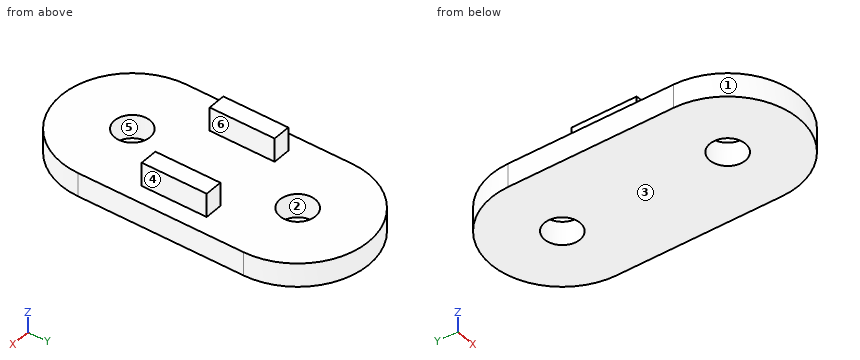
```python
from build123d import *

# Parameters (mm, degrees)
SKETCH_R     = 3
PAD_DEPTH    = 4
SKETCH001_W  = 3
SKETCH001_H  = 11
PAD001_DEPTH = 8


with BuildPart() as part:
    # Sketch → Pad (new body)
    with BuildSketch(Plane.XY):
        with BuildLine():
            ThreePointArc((12, 14), (0, 26), (-12, 14))
            Line((-12, 14), (-12, -14))
            ThreePointArc((-12, -14), (0, -26), (12, -14))
            Line((12, -14), (12, 14))
        make_face()
        with Locations((0, 14)):
            Circle(SKETCH_R, mode=Mode.SUBTRACT)
        with Locations((0, -14)):
            Circle(SKETCH_R, mode=Mode.SUBTRACT)
    extrude(amount=PAD_DEPTH)

    # Sketch001 → Pad001 (join)
    with BuildSketch(Plane.XY):
        with Locations((-7.5, 0)):
            Rectangle(SKETCH001_W, SKETCH001_H)
        with Locations((7.5, 0)):
            Rectangle(SKETCH001_W, SKETCH001_H)
    extrude(amount=PAD001_DEPTH)


solid = part.part
```
Verification items for the finished model (mm, model axes). Face numbers are marked on the shaded views. A direction names the side the tool comes from. Give positions to 0.01 mm unless a question says otherwise; leave off trailing zeros. Loops run counter-clockwise (first coordinate to the right, second up) from the corner with the lowest first, then second, coordinate; pieces in that order, holes last. Notation, with made-up numbers: M -7,18 L 39,18 A19 ccw 39,53 Z; hole C 17,73.5 d2. An arc over 180 degrees is marked long. One line per question, with ' | ' between items.
Item 1: Depth check by flat-ended pin: P1, Ø3, axis at y = -0.5, z = 6.5, coming from the -X side; P2, Ø5, axis at x = -3.5, y = 10.5, coming from the +Z side; P3, Ø3, axis at y = 13, z = 7, coming from the +X side; P4, Ø1.2, axis at y = -0.5, z = 6, coming from the +X side. Enter the tip coordinate at first touch or a pass-through.
Completed:
P1: stops at x = -9 | P2: stops at z = 4 | P3: passes through | P4: stops at x = 9
Item 2: Tool access check on the marked faces 4, 5 and 6. Record the directions out of +Z, -Z, +X, -X, +Y, -Y that give a thin tool (end or side, any length) a straight path to the whole face; none if there is none.
Completed:
face 4: +Z, +X, +Y, -Y | face 5: +Z, -Z | face 6: +Z, +Y, -Y
Item 3: Section check A-A, the plane z = 6. Record the cut outline in (x, y), plus the area to 3 significant figures.
Completed:
outline: M -9,-5.5 L -6,-5.5 L -6,5.5 L -9,5.5 Z; M 6,-5.5 L 9,-5.5 L 9,5.5 L 6,5.5 Z | area: 66.0 mm^2
Item 4: Thickness scan on line 1 (Y direction, x = 0, z = 2.4); line 2 (Y direction, x = 1.25, z = 2.75); line 3 (X direction, y = 2, z = 6.5). Record the ranges inside material, lowest first. Write a range as [from, to].
Completed:
line 1: y = [-26, -17], [-11, 11], [17, 26] | line 2: y = [-25.93, -16.73], [-11.27, 11.27], [16.73, 25.93] | line 3: x = [-9, -6], [6, 9]
Item 5: Section check B-B, the plane x = 0. Record the cut outline in (y, z), plus the area to 3 significant figures.
Completed:
outline: M -26,0 L -17,0 L -17,4 L -26,4 Z; M -11,0 L 11,0 L 11,4 L -11,4 Z; M 17,0 L 26,0 L 26,4 L 17,4 Z | area: 160 mm^2
Item 6: Section check C-C, the plane y = 0. Record the cut outline in (x, z).
Completed:
outline: M -12,0 L 12,0 L 12,4 L 9,4 L 9,8 L 6,8 L 6,4 L -6,4 L -6,8 L -9,8 L -9,4 L -12,4 Z
Item 7: Draft check along X on the marked faces 1, 2 and 3. Enter one of: +X half, -X half, draft (parallel to the pull), parting line (faces both ways), or undercut.
Completed:
face 1: parting line | face 2: undercut | face 3: draft
Item 8: Section check D-D, the plane y = -16. Record the cut outline in (x, z), plus the area to 3 significant figures.
Completed:
outline: M -11.83,0 L -2.24,0 L -2.24,4 L -11.83,4 Z; M 2.24,0 L 11.83,0 L 11.83,4 L 2.24,4 Z | area: 76.8 mm^2
